```python
from build123d import *

# Parameters (mm, degrees)
BOSS_EXTRUDE2_DEPTH = 18
SKETCH2_W           = 18
SKETCH2_H           = 100
CUT_EXTRUDE1_DEPTH  = 18
SKETCH3_W           = 100
SKETCH3_H           = 18
CUT_EXTRUDE2_DEPTH  = 18


with BuildPart() as part:
    # Sketch1 → Boss-Extrude2 (new body)
    with BuildSketch(Plane(origin=(0, 0, 0), x_dir=(1, 0, 0), z_dir=(0, 1, 0))):
        Polygon((-282, 292), (282, 292), (282, -292), (50, -292), (50, -310.517979904), (-50, -310.517979904), (-50, -292), (-282, -292), align=None)
    extrude(amount=BOSS_EXTRUDE2_DEPTH)

    # Sketch2 → Cut-Extrude1 (cut)
    with BuildSketch(Plane.XZ):
        with Locations((267, 0)):
            Rectangle(SKETCH2_W, SKETCH2_H)
        with Locations((-267, 0)):
            Rectangle(SKETCH2_W, SKETCH2_H)
    extrude(amount=-CUT_EXTRUDE1_DEPTH, mode=Mode.SUBTRACT)

    # Sketch3 → Cut-Extrude2 (cut)
    with BuildSketch(Plane.XZ):
        with Locations((0, -277)):
            Rectangle(SKETCH3_W, SKETCH3_H)
    extrude(amount=-CUT_EXTRUDE2_DEPTH, mode=Mode.SUBTRACT)


solid = part.part
```
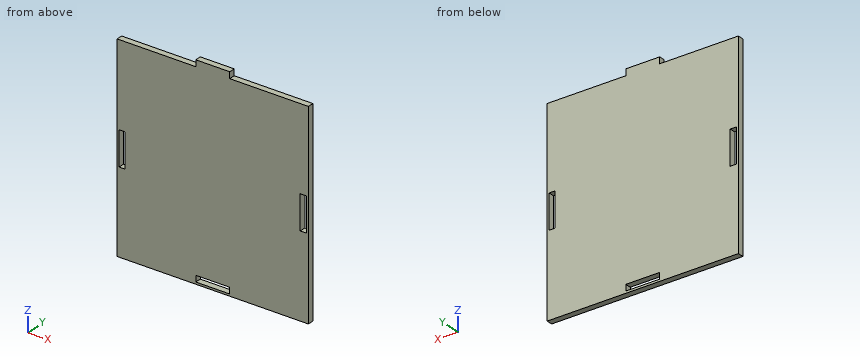
Part model, mm, in its own coordinate system. Round coordinates to 2 decimals unless told otherwise and drop trailing zeros. Write each loop counter-clockwise with the first axis right and the second up, starting at its lowest first coordinate (ties: lowest second). Pieces come first, ordered by that corner, then holes. Notation, with made-up numbers: M 30,-30 L 36,-30 A32 ccw 36,9 Z; hole C 21.5,57.25 d7. An arc over 180 degrees is marked long. Answer as CSV lines item,"result". Start each with the question number.
1) Drop flat-ended pins along their axis: pin 1 (9 mm diameter, centred on x = -265.5, y = 11, fed in from +Z); pin 2 (9 mm diameter, centred on y = 7.5, z = 303, fed in from -X). Give the stop position or say it passes through.
2) Band-saw the part on B-B (x = -42). List the corners of the cut face in (y, z).
3) Band-saw the part on C-C (y = 8.75). List the corners of the cut face in (x, z).
4) Drill centre lines: L1, parallel to X at y = 8.75, z = 21; L2, parallel to Z at x = 5, y = 6.25; L3, parallel to Z at x = -169, y = 16.75. Where is each one in solid material? Low to high.
5) Band-saw the part on A-A (z = -43). List the corners of the cut face in (x, y).
6) Band-saw the part on D-D (x = 172.5). List the corners of the cut face in (y, z).
Worked out:
1,pin 1,"z = 292"
1,pin 2,"x = -50"
2,outline,"M 0,-292 L 18,-292 L 18,-286 L 0,-286 Z; M 0,-268 L 18,-268 L 18,310.52 L 0,310.52 Z"
3,outline,"M -282,-292 L 282,-292 L 282,292 L 50,292 L 50,310.52 L -50,310.52 L -50,292 L -282,292 Z; hole M -276,-50 L -258,-50 L -258,50 L -276,50 Z; hole M -50,-286 L 50,-286 L 50,-268 L -50,-268 Z; hole M 258,-50 L 276,-50 L 276,50 L 258,50 Z"
4,L1,"-282 to -276, -258 to 258, 276 to 282"
4,L2,"-292 to -286, -268 to 310.52"
4,L3,"-292 to 292"
5,outline,"M -282,0 L -276,0 L -276,18 L -282,18 Z; M -258,0 L 258,0 L 258,18 L -258,18 Z; M 276,0 L 282,0 L 282,18 L 276,18 Z"
6,outline,"M 0,-292 L 18,-292 L 18,292 L 0,292 Z"
